Source: CAD feature listing. Evaluate the final solid. Frame: model axes, mm. Coordinates: 2 decimals unless noted, no trailing zeros. Order: outer loops, then holes, each group sorted by start corner. A loop starts at its lowest first (then second) coordinate and runs counter-clockwise, first axis right, second up. Notation, with made-up numbers: (21, 26.25) -> (78, 26.25) arc R12 cw to (78, 40.25) -> close; hole circle Ø11 at (47, -27). An arc over 180 degrees is marked (long way). Put each result on its own line as item: value.
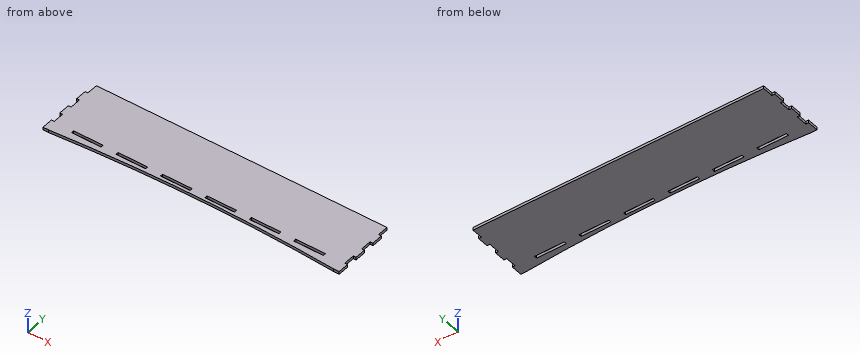
Autodesk Inventor part; units mm, degrees
ref_plane "YZ Plane" through (0, 0, 0) normal (1, 0, 0) x (0, 1, 0)
ref_plane "XZ Plane" through (0, 0, 0) normal (0, 1, 0) x (-1, 0, 0)
ref_plane "XY Plane" through (0, 0, 0) normal (0, 0, 1) x (1, 0, 0)
sketch "Sketch1" plane through (0, 0, 0) normal (0, 0, 1) x (1, 0, 0)
  line L0 (-998.1754, 340.1521) -> (1033.8246, 340.1521)
  line L1 (1033.8246, 340.1521) -> (1033.8246, -117.0479)
  line L2 (-998.1754, -117.0479) -> (-998.1754, 340.1521)
  arc A0 (995.7246, -117.0479) -> (-960.0754, -117.0479) centre (17.8246, -12647.7146) ccw
  line L3 (1033.8246, -117.0479) -> (995.7246, -117.0479)
  line L4 (-960.0754, -117.0479) -> (-998.1754, -117.0479)
  point P0 (0, 0)
  dimension "d0" = 2032
  dimension "d1" = 457.2
extrude "Extrusion1" add sketch "Sketch1" along normal blind 19.05
sketch "Sketch2" plane through (0, 0, 19.05) normal (0, 0, 1) x (1, 0, 0)
  line L0 (1033.8246, 340.1521) -> (-998.1754, 340.1521)
  line L1 (-998.1754, -117.0479) -> (-960.0754, -117.0479)
  line L2 (-998.1754, 340.1521) -> (-979.1254, 340.1521)
  line L3 (-979.1254, 340.1521) -> (-979.1254, -117.0479)
  line L4 (-979.1254, -117.0479) -> (-998.1754, -117.0479)
  line L5 (-998.1754, -117.0479) -> (-998.1754, 340.1521)
  line L6 (1033.8246, -117.0479) -> (1033.8246, 340.1521)
  line L7 (1033.8246, 340.1521) -> (1014.7746, 340.1521)
  line L8 (1014.7746, 340.1521) -> (1014.7746, -117.0479)
  line L9 (1014.7746, -117.0479) -> (1033.8246, -117.0479)
  line L10 (1033.8246, -117.0479) -> (1033.8246, 340.1521)
  line L11 (-998.1754, 340.1521) -> (-998.1754, -117.0479)
  line L12 (-998.1754, 263.9521) -> (-979.1254, 263.9521)
  line L13 (1014.7746, 263.9521) -> (1033.8246, 263.9521)
  line L14 (-998.1754, 187.7521) -> (-979.1254, 187.7521)
  line L15 (1014.7746, 187.7521) -> (1033.8246, 187.7521)
  line L16 (-998.1754, 111.5521) -> (-979.1254, 111.5521)
  line L17 (1014.7746, 111.5521) -> (1033.8246, 111.5521)
  line L18 (-998.1754, 35.3521) -> (-979.1254, 35.3521)
  line L19 (1014.7746, 35.3521) -> (1033.8246, 35.3521)
  line L20 (1033.8246, -40.8479) -> (1014.7746, -40.8479)
  line L21 (-979.1254, -40.8479) -> (-998.1754, -40.8479)
  point P0 (0, 0)
  dimension "d7" = 19.05
  dimension "d8" = 19.05
extrude "Extrusion2" cut sketch "Sketch2" against normal blind 19.05 contours L6 L13 L8 L0 | L3 L12 L5 L0 | L6 L17 L8 L15 | L3 L16 L5 L14 | L6 L20 L8 L19 | L3 L21 L5 L18
sketch "Sketch4" plane through (0, 0, 19.05) normal (0, 0, 1) x (1, 0, 0)
  line L0 (-845.7754, -40.8479) -> (-845.7754, -59.8979)
  line L1 (-998.1754, 111.5521) -> (-998.1754, 35.3521)
  line L2 (-642.5754, -40.8479) -> (-642.5754, -59.8979)
  line L3 (-540.9754, -40.8479) -> (-540.9754, -59.8979)
  line L4 (-337.7754, -40.8479) -> (-337.7754, -59.8979)
  line L5 (-236.1754, -40.8479) -> (-236.1754, -59.8979)
  line L6 (-32.9754, -40.8479) -> (-32.9754, -59.8979)
  line L7 (68.6246, -40.8479) -> (68.6246, -59.8267)
  line L8 (271.8246, -40.8479) -> (271.8246, -59.8267)
  line L9 (373.4246, -40.8479) -> (373.4246, -59.8979)
  line L10 (576.6246, -40.8479) -> (576.6246, -59.8979)
  line L11 (678.2246, -40.8479) -> (678.2246, -59.8979)
  line L12 (881.4246, -40.8479) -> (881.4246, -59.8979)
  arc A0 (995.7246, -117.0479) -> (-960.0754, -117.0479) centre (17.8246, -12647.7146) ccw
  line L13 (-998.1754, -40.8479) -> (-998.1754, -117.0479)
  line L14 (1014.7746, 340.1521) -> (-979.1254, 340.1521)
  line L15 (1014.7746, 340.1521) -> (1014.7746, 263.9521)
  line L16 (-979.1254, 340.1521) -> (1014.7746, 340.1521)
  line L17 (-845.7754, -40.8479) -> (-642.5754, -40.8479)
  line L18 (-845.7754, -59.8979) -> (-642.5754, -59.8979)
  line L19 (-540.9754, -59.8979) -> (-337.7754, -59.8979)
  line L20 (-540.9754, -40.8479) -> (-337.7754, -40.8479)
  line L21 (-236.1754, -40.8479) -> (-32.9754, -40.8479)
  line L22 (68.6246, -40.8479) -> (271.8246, -40.8479)
  line L23 (373.4246, -59.8979) -> (576.6246, -59.8979)
  line L24 (678.2246, -59.8979) -> (881.4246, -59.8979)
  line L25 (373.4246, -40.8479) -> (576.6246, -40.8479)
  line L26 (678.2246, -40.8479) -> (881.4246, -40.8479)
  line L27 (-236.1754, -59.8979) -> (-32.9754, -59.8979)
  line L28 (68.6246, -59.8267) -> (271.8246, -59.8267)
  point P0 (0, 0)
  dimension "d18" = 152.4
  dimension "d19" = 203.2
  dimension "d26" = 457.2
  dimension "d27" = 203.2
  dimension "d28" = 101.6
  dimension "d29" = 203.2
  dimension "d30" = 101.6
  dimension "d31" = 101.6
  dimension "d32" = 101.6
  dimension "d33" = 203.2
  dimension "d34" = 203.2
  dimension "d35" = 203.2
extrude "Extrusion4" cut sketch "Sketch4" against normal blind 25.4
properties part number "back" material "Wood (Birch)"
1. Cut plane A-A on x = -389. Output: boundary loops of the cut face in (y, z).
Numbers:
outline: (-85.53, 0) -> (-59.9, 0) -> (-59.9, 19.05) -> (-85.53, 19.05) -> close; (-40.85, 0) -> (340.15, 0) -> (340.15, 19.05) -> (-40.85, 19.05) -> close
2. Cut plane C-C on y = 287. Output: boundary loops of the cut face in (x, z), plus the area to 3 significant figures.
Numbers:
outline: (-979.13, 0) -> (1014.77, 0) -> (1014.77, 19.05) -> (-979.13, 19.05) -> close
area: 38,000 mm2
3. First-contact query: pin 1 (5.5 mm diameter, centred on y = 305, z = 8, fed in from -X); pin 2 (5.5 mm diameter, centred on x = -985, z = 14, fed in from +Y); pin 3 (12 mm diameter, centred on x = -755, y = -27.5, fed in from -Z). Flat tips, straight axial feed; report the tip coordinate or a pass-through.
Numbers:
pin 1: stops at x = -979.13
pin 2: stops at y = 263.95
pin 3: stops at z = 0
4. Cut plane B-B on z = 12.25. Count the separate pieces of the cut face and the enclosed holes in it, plus the area to 3 significant figures.
Numbers:
separate pieces: 1
enclosed holes: 6
area: 847,000 mm2
5. Cut plane D-D on x = -790. Output: boundary loops of the cut face in (y, z).
Numbers:
outline: (-104.94, 0) -> (-59.9, 0) -> (-59.9, 19.05) -> (-104.94, 19.05) -> close; (-40.85, 0) -> (340.15, 0) -> (340.15, 19.05) -> (-40.85, 19.05) -> close
6. Ray query, line 1 along Y through (x, z) = (84, 2.75); line 2 along Y through (x, z) = (-446, 15); line 3 along X through (y, z) = (18.5, 6). Return the intervals inside material, ascending.
Numbers:
line 1: y = -79.12 to -59.83, -40.85 to 340.15
line 2: y = -87.51 to -59.9, -40.85 to 340.15
line 3: x = -979.13 to 1014.77
